For this review, take the finished solid that the model builds, in its own axes (mm). A direction names the side the tool comes from. Coordinates: 2 decimals unless noted, no trailing zeros. Loops run counter-clockwise (first coordinate to the right, second up) from the corner with the lowest first, then second, coordinate; pieces in that order, holes last. Notation, with made-up numbers: (54.25, 39) - (95.25, 39) arc R24 ccw to (95.25, 64) - close; hole circle Ø4 at (-37.5, 38). An arc over 180 degrees is marked (long way). Answer as a JSON object with one key per item and string values. Group by question number.
Item 1: We need section B-B (z = -36). Give the boundary of the cut face in (x, y).
Item 2: Tool access review of faces 5 (the cylindrical face through (90.61, 28.53, 57.06)), 6 (the cylindrical face through (283.83, 0.75, 25.04)), 7 (the flat face through (15, -32, 14.224)): name each direction out of +Z, -Z, +X, -X, +Y, -Y from which nothing blocks a thin tool from reaching the whole face with its end or side.
Item 3: We need section A-A (x = -266.7). Give the boundary of the cut face in (y, z) (3 decimals).
Item 4: Clearance check with flat-ended pins moving along their axes: pin 1 (5 mm diameter, centred on x = 147, z = 35, fed in from -Y); pin 2 (1 mm diameter, centred on y = -14, z = 49, fed in from -X); pin 3 (8 mm diameter, centred on x = -28.5, z = 27, fed in from +Y). State where each tip first meets the part, or that it passes through.
Item 5: We need section C-C (x = 349.5). Give the boundary of the cut face in (y, z).
Item 6: Mouldability with a two-part tool opening along Y and no side actions: class faces 1 (the flat face through (-232.9, -82.6, 25)), 2 (the flat face through (-229.28, 83.17, 25.04)), 3 (the cylindrical face through (-268.93, 17, 25.04)), 4 (the cylindrical face through (72.44, 22.81, 47.85)) as released by +Y, released by -Y, zero draft, split by the parting line, or undercut.
Item 7: To check wall thickness, follow line 1 (Z direction, x = 2, y = -175); line 2 (Y direction, x = 317.5, z = 34.5) (3 decimals); line 3 (Y direction, x = 218, z = 13.5). State the ranges of each line that lie inside material, in increasing order.
from build123d import *

# Parameters (mm, degrees)
F0_R     = 17.145
F1_DEPTH = 50.8
F2_R     = 94.996
F2_R_2   = 75.946
F3_DEPTH = 12.7
F4_R     = 75.946
F5_DEPTH = 31.75
F6_R     = 113.03
F6_R_2   = 69.85
F7_DEPTH = 61.976
F8_R     = 69.85
F9_DEPTH = 76.2


with BuildPart() as f1:
    # F0 (on Top) → F1 (new body)
    with BuildSketch(Plane.XY):
        with BuildLine():
            ThreePointArc((34.925, 0), (-24.695704, -24.695704), (0, 34.925))
            Line((0, 34.925), (0, 198.755))
            ThreePointArc((0, 198.755), (-17.145, 215.9), (0, 233.045))
            Line((0, 233.045), (0, 249.555))
            ThreePointArc((0, 249.555), (-17.145, 266.7), (0, 283.845))
            Line((0, 283.845), (0, 300.355))
            ThreePointArc((0, 300.355), (-17.145, 317.5), (0, 334.645))
            Line((0, 334.645), (0, 412.712916))
            ThreePointArc((0, 412.712916), (-41.261016, 397.480696), (-62.726854, 359.091769))
            Line((-62.726854, 359.091769), (-103.050756, 103.050756))
            Line((-103.050756, 103.050756), (-359.091769, 62.726854))
            ThreePointArc((-359.091769, 62.726854), (-397.480696, 41.261016), (-412.712916, 0))
            ThreePointArc((-412.712916, 0), (-397.480696, -41.261016), (-359.091769, -62.726854))
            Line((-359.091769, -62.726854), (-103.050756, -103.050756))
            Line((-103.050756, -103.050756), (-62.726854, -359.091769))
            ThreePointArc((-62.726854, -359.091769), (-41.261016, -397.480696), (0, -412.712916))
            ThreePointArc((0, -412.712916), (41.261016, -397.480696), (62.726854, -359.091769))
            Line((62.726854, -359.091769), (103.050756, -103.050756))
            Line((103.050756, -103.050756), (359.091769, -62.726854))
            ThreePointArc((359.091769, -62.726854), (397.480696, -41.261016), (412.712916, 0))
            Line((412.712916, 0), (334.645, 0))
            ThreePointArc((334.645, 0), (317.5, -17.145), (300.355, 0))
            Line((300.355, 0), (283.845, 0))
            ThreePointArc((283.845, 0), (266.7, -17.145), (249.555, 0))
            Line((249.555, 0), (233.045, 0))
            ThreePointArc((233.045, 0), (215.9, -17.145), (198.755, 0))
            Line((198.755, 0), (34.925, 0))
        make_face()
        with Locations((0, -317.5)):
            Circle(F0_R, mode=Mode.SUBTRACT)
        with Locations((0, -266.7)):
            Circle(F0_R, mode=Mode.SUBTRACT)
        with Locations((0, -215.9)):
            Circle(F0_R, mode=Mode.SUBTRACT)
        with Locations((-317.5, 0)):
            Circle(F0_R, mode=Mode.SUBTRACT)
        with Locations((-266.7, 0)):
            Circle(F0_R, mode=Mode.SUBTRACT)
        with Locations((-215.9, 0)):
            Circle(F0_R, mode=Mode.SUBTRACT)
        with BuildLine():
            Line((0, 198.755), (0, 34.925))
            ThreePointArc((0, 34.925), (13.365219, 32.266493), (24.695704, 24.695704))
            Line((24.695704, 24.695704), (103.050756, 103.050756))
            Line((103.050756, 103.050756), (62.726854, 359.091769))
            ThreePointArc((62.726854, 359.091769), (41.261016, 397.480696), (0, 412.712916))
            Line((0, 412.712916), (0, 334.645))
            ThreePointArc((0, 334.645), (12.123346, 329.623346), (17.145, 317.5))
            ThreePointArc((17.145, 317.5), (12.123346, 305.376654), (0, 300.355))
            Line((0, 300.355), (0, 283.845))
            ThreePointArc((0, 283.845), (12.123346, 278.823346), (17.145, 266.7))
            ThreePointArc((17.145, 266.7), (12.123346, 254.576654), (0, 249.555))
            Line((0, 249.555), (0, 233.045))
            ThreePointArc((0, 233.045), (12.123346, 228.023346), (17.145, 215.9))
            ThreePointArc((17.145, 215.9), (12.123346, 203.776654), (0, 198.755))
        make_face()
        with BuildLine():
            Line((103.050756, 103.050756), (24.695704, 24.695704))
            ThreePointArc((24.695704, 24.695704), (32.266493, 13.365219), (34.925, 0))
            Line((34.925, 0), (198.755, 0))
            ThreePointArc((198.755, 0), (215.9, 17.145), (233.045, 0))
            Line((233.045, 0), (249.555, 0))
            ThreePointArc((249.555, 0), (266.7, 17.145), (283.845, 0))
            Line((283.845, 0), (300.355, 0))
            ThreePointArc((300.355, 0), (317.5, 17.145), (334.645, 0))
            Line((334.645, 0), (412.712916, 0))
            ThreePointArc((412.712916, 0), (397.480696, 41.261016), (359.091769, 62.726854))
            Line((359.091769, 62.726854), (103.050756, 103.050756))
        make_face()
    extrude(amount=F1_DEPTH)

    # F2 (on face) → F3 (join)
    with BuildSketch(Plane.XY.offset(50.8)):
        Circle(F2_R)
        Circle(F2_R_2, mode=Mode.SUBTRACT)
    extrude(amount=F3_DEPTH)

    # F4 (on face) → F5 (cut)
    with BuildSketch(Plane.XY.offset(63.5)):
        Circle(F4_R)
    extrude(amount=-F5_DEPTH, mode=Mode.SUBTRACT)

    # F6 (on face) → F7 (join)
    with BuildSketch(Plane(origin=(0, 0, 0), x_dir=(1, 0, 0), z_dir=(0, 0, -1))):
        Circle(F6_R)
        Circle(F6_R_2, mode=Mode.SUBTRACT)
    extrude(amount=F7_DEPTH)

    # F8 (on face) → F9 (cut)
    with BuildSketch(Plane(origin=(0, 0, -61.976), x_dir=(1, 0, 0), z_dir=(0, 0, -1))):
        Circle(F8_R)
    extrude(amount=-F9_DEPTH, mode=Mode.SUBTRACT)


solid = f1.part
Check sheet entries:
{
 "1": {"outline": "circle Ø226.06 at (0, 0); hole circle Ø139.7 at (0, 0)"},
 "2": {"face 5": "+Z", "face 6": "+Z, -Z", "face 7": "-Z"},
 "3": {"outline": "(-77.278, 0) - (-17.145, 0) - (-17.145, 50.8) - (-77.278, 50.8) - close; (17.145, 0) - (77.278, 0) - (77.278, 50.8) - (17.145, 50.8) - close"},
 "4": {"pin 1": "stops at y = -96.52", "pin 2": "stops at x = -411.26", "pin 3": "stops at y = 407.8"},
 "5": {"outline": "(-64.24, 0) - (64.24, 0) - (64.24, 50.8) - (-64.24, 50.8) - close"},
 "6": {"face 1": "released by -Y", "face 2": "released by +Y", "face 3": "undercut", "face 4": "undercut"},
 "7": {"line 1": "z = 0 to 50.8", "line 2": "y = -69.277 to -17.145, 17.145 to 69.277", "line 3": "y = -84.95 to -17.02, 17.02 to 84.95"}
}
